The model under review builds one solid part; all positions refer to its coordinate system, in mm. Give positions to 0.01 mm unless a question says otherwise; leave off trailing zeros. Loops run counter-clockwise (first coordinate to the right, second up) from the corner with the lowest first, then second, coordinate; pieces in that order, holes last. Notation, with made-up numbers: M 82,34 L 130,34 A31 cw 130,65 Z; hole C 15.5,26.5 d7. An arc over 180 degrees is marked long. One line per item, written item: value. Start each with the question number.
Q1. We need section B-B on x = 224.5. Write out the cut boundary in (y, z), plus the area to 3 significant figures.
Q2. To check wall thickness, follow line 1 along Z through (x, y) = (175, 0.8); line 2 along Z through (x, y) = (233, 0.8); line 3 along Z through (x, y) = (220, 1.25). State the ranges of each line that lie inside material, in increasing order. Write a range as from..to.
Q3. We need section A-A on y = -1.45. Give the number of separate pieces and of enclosed holes in the cut face, plus the area to 3 significant figures.
```python
from build123d import *

# Parameters (mm, degrees)
BOSS_EXTRUDE1_DEPTH = 272
SKETCH2_R           = 1
CUT_EXTRUDE1_DEPTH  = 5.8


with BuildPart() as part:
    # Sketch1 → Boss-Extrude1 (new body)
    with BuildSketch(Plane(origin=(0, 0, 0), x_dir=(0, 0, -1), z_dir=(1, 0, 0))):
        with BuildLine():
            Line((3.5, 2.4), (-3.5, 2.4))
            Line((-3.5, 2.4), (-3.5, 1.4))
            ThreePointArc((-3.5, 1.4), (-3.146446609, 1.253553391), (-3, 0.9))
            ThreePointArc((-3, 0.9), (-3.146446609, 0.546446609), (-3.5, 0.4))
            Line((-3.5, 0.4), (-3.5, -2.4))
            Line((-3.5, -2.4), (3.5, -2.4))
            Line((3.5, -2.4), (3.5, 0.4))
            ThreePointArc((3.5, 0.4), (3, 0.9), (3.5, 1.4))
            Line((3.5, 1.4), (3.5, 2.4))
        make_face()
    extrude(amount=BOSS_EXTRUDE1_DEPTH)

    # Sketch2 → Cut-Extrude1 (cut, through all)
    with BuildSketch(Plane(origin=(0, 2.4, 0), x_dir=(1, 0, 0), z_dir=(0, 1, 0))):
        with Locations((10, 0)):
            Circle(SKETCH2_R)
        with Locations((25, 0)):
            Circle(SKETCH2_R)
        with Locations((40, 0)):
            Circle(SKETCH2_R)
        with Locations((55, 0)):
            Circle(SKETCH2_R)
        with Locations((70, 0)):
            Circle(SKETCH2_R)
        with Locations((85, 0)):
            Circle(SKETCH2_R)
        with Locations((100, 0)):
            Circle(SKETCH2_R)
        with Locations((115, 0)):
            Circle(SKETCH2_R)
        with Locations((130, 0)):
            Circle(SKETCH2_R)
        with Locations((145, 0)):
            Circle(SKETCH2_R)
        with Locations((160, 0)):
            Circle(SKETCH2_R)
        with Locations((175, 0)):
            Circle(SKETCH2_R)
        with Locations((190, 0)):
            Circle(SKETCH2_R)
        with Locations((205, 0)):
            Circle(SKETCH2_R)
        with Locations((220, 0)):
            Circle(SKETCH2_R)
        with Locations((235, 0)):
            Circle(SKETCH2_R)
        with Locations((250, 0)):
            Circle(SKETCH2_R)
        with Locations((265, 0)):
            Circle(SKETCH2_R)
        with Locations((280, 0)):
            Circle(SKETCH2_R)
        with Locations((295, 0)):
            Circle(SKETCH2_R)
        with Locations((310, 0)):
            Circle(SKETCH2_R)
        with Locations((325, 0)):
            Circle(SKETCH2_R)
        with Locations((340, 0)):
            Circle(SKETCH2_R)
        with Locations((355, 0)):
            Circle(SKETCH2_R)
        with Locations((370, 0)):
            Circle(SKETCH2_R)
        with Locations((385, 0)):
            Circle(SKETCH2_R)
        with Locations((400, 0)):
            Circle(SKETCH2_R)
        with Locations((415, 0)):
            Circle(SKETCH2_R)
        with Locations((430, 0)):
            Circle(SKETCH2_R)
        with Locations((445, 0)):
            Circle(SKETCH2_R)
        with Locations((460, 0)):
            Circle(SKETCH2_R)
    extrude(amount=-CUT_EXTRUDE1_DEPTH, mode=Mode.SUBTRACT)


solid = part.part
```
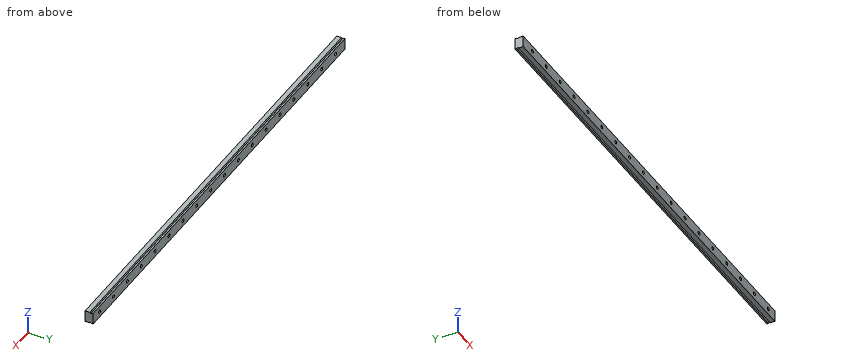
Solved:
1. outline: M -2.4,-3.5 L 0.4,-3.5 A0.5 cw 1.4,-3.5 L 2.4,-3.5 L 2.4,3.5 L 1.4,3.5 A0.5 cw 0.4,3.5 L -2.4,3.5 Z
1. area: 32.8 mm2
2. line 1: -3.01..-1, 1..3.01
2. line 2: -3.01..3.01
2. line 3: -3.14..-1, 1..3.14
3. separate pieces: 1
3. enclosed holes: 18
3. area: 1,850 mm2
